Can you work these out from the model? Positions are in its coordinate system, mm. A direction names the side the tool comes from. Round coordinates to 2 decimals unless told otherwise and drop trailing zeros. Write each loop counter-clockwise with the first axis right and the second up, starting at its lowest first coordinate (ties: lowest second). Pieces come first, ordered by that corner, then holes. Notation, with made-up numbers: (-2, -32) -> (46, -32) arc R16 cw to (46, -4) -> close; hole circle Ø6 at (75.25, 48). An arc over 180 degrees is marked (long way). Write item = value, one per line. Start each with the question number.
1) If I drill on line 1 (X direction, y = -0.25, z = -5.5); line 2 (X direction, y = -1.5, z = -1.5); line 3 (Z direction, x = 15.5, y = -1.5), over which ranges is the centre line in solid material (lowest first)?
2) Imagine slicing it at C-C, the plane x = 14.5. Please give me the cut outline in (y, z), then the cut area to 3 significant figures.
3) For faces 1 (the face through (-1.61, -1.85, -4.47)), 2 (the face through (-36, -1, 6.189)), 3 (the face through (40, 5, 6.855)), 4 (the face through (-36, -1, -6.189)), 5 (the face through (-42.74, 0.14, 0.09)), which set-ups out of +Z, -Z, +X, -X, +Y, -Y let a thin tool reach every point of the face, with its end or its side?
4) Thinking about a two-plate mould opening in X: for faces 6 (the face through (40, 5, -6.855)), 7 (the face through (-44.35, 0.21, -0.09)), which applies, +X half, -X half, draft (parallel to the pull), parting line (faces both ways), or undercut?
5) Imagine slicing it at A-A, the plane y = 0. Please give me the cut outline in (x, z), then the cut area to 3 significant figures.
6) Imagine slicing it at D-D, the plane z = -4. Please give me the cut outline in (x, y), then the cut area to 3 significant figures.
7) Imagine slicing it at B-B, the plane z = -0.75. Please give me the cut outline in (x, y), then the cut area to 3 significant figures.
8) I'm going to push flat-ended pins straight in: pin 1 (3 mm diameter, centred on x = 29.5, y = 4.5, fed in from +Z); pin 2 (3 mm diameter, centred on x = -16, y = 2.5, fed in from +Z); pin 3 (3 mm diameter, centred on y = 4, z = 0, fed in from +X). Where does each tip first touch, or does it pass through?
from build123d import *

# Parameters (mm, degrees)
SKETCH1_R                = 4.8387
BOSS_EXTRUDE1_DEPTH      = 39.51605
BOSS_EXTRUDE1_DEPTH_BACK = 39.51605
SKETCH2_R                = 4.8387
BOSS_EXTRUDE2_DEPTH      = 6.18871
BOSS_EXTRUDE2_DEPTH_BACK = 6.18871
SKETCH3_R                = 3.2258
CUT_EXTRUDE1_DEPTH       = 13.37742
SKETCH4_R                = 6.4516
BOSS_EXTRUDE3_DEPTH      = 6.85546
BOSS_EXTRUDE3_DEPTH_BACK = 6.85546
SKETCH5_R                = 4.8387
CUT_EXTRUDE2_DEPTH       = 14.7109201


with BuildPart() as part:
    # Sketch1 → Boss-Extrude1 (new body, two sides)
    with BuildSketch(Plane(origin=(0, 0, 0), x_dir=(0, 0, -1), z_dir=(1, 0, 0))) as boss_extrude1_sk:
        Circle(SKETCH1_R)
    extrude(amount=BOSS_EXTRUDE1_DEPTH)
    extrude(boss_extrude1_sk.sketch, amount=-BOSS_EXTRUDE1_DEPTH_BACK)

    # Sketch2 → Boss-Extrude2 (add, two sides)
    with BuildSketch(Plane.XY) as boss_extrude2_sk:
        with Locations((-39.51605, 0)):
            Circle(SKETCH2_R)
    extrude(amount=BOSS_EXTRUDE2_DEPTH)
    extrude(boss_extrude2_sk.sketch, amount=-BOSS_EXTRUDE2_DEPTH_BACK)

    # Sketch3 → Cut-Extrude1 (cut, through all)
    with BuildSketch(Plane.XY.offset(6.18871)):
        with Locations((-39.51605, 0)):
            Circle(SKETCH3_R)
    extrude(amount=-CUT_EXTRUDE1_DEPTH, mode=Mode.SUBTRACT)

    # Sketch4 → Boss-Extrude3 (add, two sides)
    with BuildSketch(Plane.XY) as boss_extrude3_sk:
        with Locations((39.51605, 0)):
            Circle(SKETCH4_R)
    extrude(amount=BOSS_EXTRUDE3_DEPTH)
    extrude(boss_extrude3_sk.sketch, amount=-BOSS_EXTRUDE3_DEPTH_BACK)

    # Sketch5 → Cut-Extrude2 (cut, through all)
    with BuildSketch(Plane.XY.offset(6.85546)):
        with Locations((39.51605, 0)):
            Circle(SKETCH5_R)
    extrude(amount=-CUT_EXTRUDE2_DEPTH, mode=Mode.SUBTRACT)


solid = part.part
Reported:
q1.line_1 = -44.35 to -42.73, -36.3 to -34.68, 33.07 to 34.68, 44.35 to 45.96
q1.line_2 = -44.12 to -42.37, -36.66 to 34.92, 44.12 to 45.79
q1.line_3 = -4.6 to 4.6
q2.outline = circle Ø9.68 at (0, 0)
q2.area = 73.6 mm²
q3.face_1 = none
q3.face_2 = +Z, -X, +Y, -Y
q3.face_3 = +Z, +X, -X, +Y, -Y
q3.face_4 = -Z, -X, +Y, -Y
q3.face_5 = +Z, -Z
q4.face_6 = draft
q4.face_7 = undercut
q5.outline = (-44.35, -6.19) -> (-42.74, -6.19) -> (-42.74, 6.19) -> (-44.35, 6.19) -> close; (-36.29, -6.19) -> (-34.68, -6.19) -> (-34.68, -4.84) -> (33.06, -4.84) -> (33.06, -6.86) -> (34.68, -6.86) -> (34.68, 6.86) -> (33.06, 6.86) -> (33.06, 4.84) -> (-34.68, 4.84) -> (-34.68, 6.19) -> (-36.29, 6.19) -> close; (44.35, -6.86) -> (45.97, -6.86) -> (45.97, 6.86) -> (44.35, 6.86) -> close
q5.area = 740 mm²
q6.outline = (-35.52, -2.72) -> (33.67, -2.72) arc R6.45 ccw (long way) to (33.67, 2.72) -> (-35.52, 2.72) arc R4.84 ccw (long way) to start; hole circle Ø6.45 at (-39.52, 0); hole circle Ø9.68 at (39.52, 0)
q6.area = 469 mm²
q7.outline = (-38.77, -4.78) -> (35.18, -4.78) arc R6.45 ccw (long way) to (35.18, 4.78) -> (-38.77, 4.78) arc R4.84 ccw (long way) to start; hole circle Ø6.45 at (-39.52, 0); hole circle Ø9.68 at (39.52, 0)
q7.area = 761 mm²
q8.pin_1 = 3.8
q8.pin_2 = 4.73
q8.pin_3 = 45.46
